Autodesk Inventor part; units mm, degrees
ref_plane "YZ Plane" through (0, 0, 0) normal (1, 0, 0) x (0, 1, 0)
ref_plane "XZ Plane" through (0, 0, 0) normal (0, 1, 0) x (-1, 0, 0)
ref_plane "XY Plane" through (0, 0, 0) normal (0, 0, 1) x (1, 0, 0)
sketch "Skizze1" plane through (0, 0, 0) normal (0, 1, 0) x (-1, 0, 0)
  circle A0 centre (0, 0) radius 8.65
  circle A1 centre (0, 0) radius 15
  dimension "d0" = 17.3
  dimension "d1" = 30
extrude "Extrusion1" add sketch "Skizze1" along normal blind 30
sketch "Skizze2" plane through (0, 0, 0) normal (1, 0, 0) x (0, 1, 0)
  line L0 (30, -15) -> (30, 15)
  line L1 (0, -15) -> (0, 15)
  circle A0 centre (3.817, 0) radius 1.4
  point P0 (0, 0)
  dimension "d4" = 2.8
extrude "Extrusion2" cut sketch "Skizze2" against normal blind 20
pattern_circular "Runde Anordnung1" count 3 over 360 about axis through (0, 0, 0) along (0, 1, 0) of "Extrusion2"
sketch "Skizze3" plane through (0, 30, 0) normal (0, 1, 0) x (1, 0, 0)
  circle A0 centre (0, 0) radius 15
  circle A1 centre (0, 0) radius 15
  arc A2 (-14.368, 4.3081) -> (-15, 0) centre (-12.5959, 1.8477) ccw
  point P0 (-15, 0)
  point P1 (-14.368, 4.3081)
extrude "Extrusion3" add sketch "Skizze3" against normal up to surface (30 mm away) contours A0 A2
pattern_circular "Runde Anordnung2" count 22 over 360 about axis through (0, 0, 0) along (0, 1, 0) of "Extrusion3"
properties part number "00_CCTV_Lens_Knob"
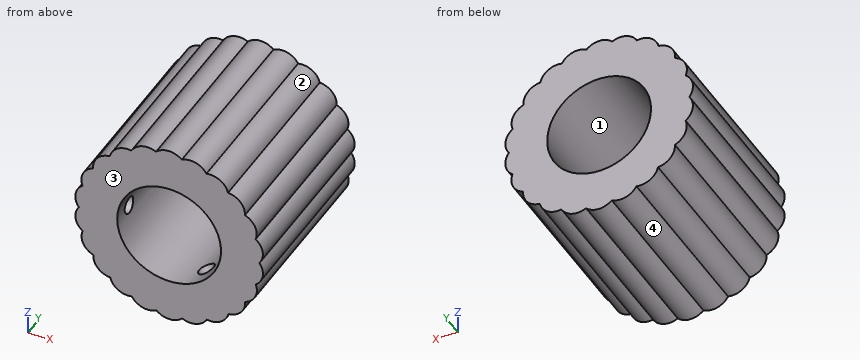
Check sheet for the modelled part. Datum: model origin and axes. Units: mm. Face numbers are marked on the shaded views. Give positions to 0.01 mm unless a question says otherwise; leave off trailing zeros. Order: outer loops, then holes, each group sorted by start corner. A loop starts at its lowest first (then second) coordinate and runs counter-clockwise, first axis right, second up. Notation, with made-up numbers: M 28,23 L 73,23 A11 cw 73,36 Z; hole C 48.5,10.5 d3. An arc over 180 degrees is marked long. Answer in a Markdown table with one row per item.
1) Release check for a two-part mould opening along Z. For the marked faces 1, 2, 3 and 4 record: +Z half, -Z half, draft (parallel to the pull), parting line (faces both ways), or undercut.
Filled sheet:
| item | result |
|---|---|
| face 1 | undercut |
| face 2 | +Z half |
| face 3 | draft |
| face 4 | -Z half |
2) Cross-section at A-A, the plane z = 3. Enter the section's corners in (x, y).
Filled sheet:
| item | result |
|---|---|
| outline | M -15.38,0 L -8.11,0 L -8.11,30 L -15.38,30 Z; M 8.11,0 L 15.4,0 L 15.4,30 L 8.11,30 Z |
3) Thickness scan on L1, parallel to Y at x = -10.5, z = 0; L2, parallel to Z at x = 0, y = 19; L3, parallel to X at y = 16.5, z = -1. Record the ranges inside material, lowest first. Write a range as [from, to].
Filled sheet:
| item | result |
|---|---|
| L1 | y = [0, 2.42], [5.22, 30] |
| L2 | z = [-15.76, -8.65], [8.65, 15.76] |
| L3 | x = [-15.51, -8.59], [8.59, 15.54] |
4) Cross-section at B-B, the plane y = 24.5. Enter the section's corners in (x, z).
Filled sheet:
| item | result |
|---|---|
| outline | M -15.03,-0.04 A3.03 ccw -14.41,-4.28 A3.03 ccw -12.62,-8.16 A3.03 ccw -9.81,-11.39 A3.03 ccw -6.21,-13.69 A3.03 ccw -2.1,-14.89 A3.03 ccw 2.18,-14.87 A3.03 ccw 6.28,-13.66 A3.03 ccw 9.88,-11.33 A3.03 ccw 12.67,-8.09 A3.03 ccw 14.44,-4.19 A3.03 ccw 15.03,0.04 A3.03 ccw 14.41,4.28 A3.03 ccw 12.62,8.16 A3.03 ccw 9.81,11.39 A3.03 ccw 6.21,13.69 A3.03 ccw 2.1,14.89 A3.03 ccw -2.18,14.87 A3.03 ccw -6.28,13.66 A3.03 ccw -9.88,11.33 A3.03 ccw -12.67,8.09 A3.03 ccw -14.44,4.19 A3.03 ccw Z; hole C 0,0 d17.3 |
5) Cross-section at C-C, the plane x = 0. Enter the section's corners in (y, z).
Filled sheet:
| item | result |
|---|---|
| outline | M 0,-15.76 L 30,-15.76 L 30,-8.65 L 0,-8.65 Z; M 0,8.65 L 30,8.65 L 30,15.76 L 0,15.76 Z |
6) Gauge pin test, flat ends, axial feed: P1, Ø5, axis at x = 4, y = 18.5, coming from the +Z side; P2, Ø12, axis at x = 10, y = 14, coming from the -Z side; P3, Ø4, axis at y = 27, z = 3, coming from the +X side. Record the tip position at first contact, or that the pin passes through.
Filled sheet:
| item | result |
|---|---|
| P1 | stops at z = 15.34 |
| P2 | stops at z = -15.21 |
| P3 | stops at x = 15.63 |
7) Cross-section at D-D, the plane x = -12. Enter the section's corners in (y, z), plus the area to 3 significant figures.
Filled sheet:
| item | result |
|---|---|
| outline | M 0,-10.21 L 30,-10.21 L 30,10.22 L 0,10.22 Z; hole C 3.82,0 d2.8 |
| area | 607 mm2 |
